Part model, mm, in its own coordinate system. A direction names the side the tool comes from. Round coordinates to 2 decimals unless told otherwise and drop trailing zeros. Write each loop counter-clockwise with the first axis right and the second up, starting at its lowest first coordinate (ties: lowest second). Pieces come first, ordered by that corner, then holes. Notation, with made-up numbers: M -19.75,10 L 17.25,10 A12 cw 17.25,15 Z; hole C -32.5,35.25 d8. An arc over 180 degrees is marked long. One line per question, with ' | ' between items. Start each with the question number.
1) Saw through at C-C (z = -25). List the corners of the cut face in (x, y).
2) Saw through at A-A (z = 26). List the corners of the cut face in (x, y).
3) Wall check: probe 1 along Z at (x, y) = (2.2, 122); probe 2 along Z at (x, y) = (3.35, -122); probe 3 along Y at (x, z) = (4.1, 38.71). Give the ranges that are in metal, low to high. Write a range as [from, to].
4) Drop flat-ended pins along their axis: pin 1 Ø3 at (x, z) = (3, 23.5) entering from +Y; pin 2 Ø1.5 at (x, y) = (0.5, -40) entering from -Z; pin 3 Ø1.8 at (x, z) = (2, -54.5) entering from -Y. Give the stop position or say it passes through.
5) Tool access for faces 4 (the face through (3, 13, -29.205)), 5 (the face through (3, 119, 47)), 6 (the face through (3, 89, -53)): list every direction of +Z, -Z, +X, -X, +Y, -Y with a clear straight run to the whole face (end or side of a thin tool).
6) Saw through at B-B (x = 3.35). Give the number of separate pieces and of enclosed holes in the cut face, plus the area to 3 significant figures.
7) Mould opens along Z. For faces 1 (the face through (3, -69, -53)), 2 (the face through (3, -49, -50.29)), 3 (the face through (3, -122, -6)) say: pulls with the +Z half, pulls with the -Z half, needs draft (parallel to the pull), parting line crosses it, or undercut.
8) Saw through at D-D (y = 98). List the corners of the cut face in (x, z).
```python
from build123d import *

# Parameters (mm, degrees)
ESQUISSE1_W             = 100.58
ESQUISSE1_H             = 238
ESQUISSE1_W_2           = 10
ESQUISSE1_H_2           = 6
ESQUISSE1_W_3           = 15
BOSS_EXTRU_1_DEPTH      = 6
ESQUISSE3_W             = 20
ESQUISSE3_H             = 6
ESQUISSE3_W_2           = 6
ESQUISSE3_H_2           = 20
ESQUISSE3_W_3           = 10
BOSS_EXTRU_5_DEPTH      = 6
ESQUISSE7_W             = 6.88
ESQUISSE7_H             = 7
ENL_V_MAT_EXTRU_3_DEPTH = 6
ESQUISSE8_R             = 1.5
ENL_V_MAT_EXTRU_4_DEPTH = 6


with BuildPart() as part:
    # Esquisse1 → Boss.-Extru.1 (new body)
    with BuildSketch(Plane(origin=(0, 0, 0), x_dir=(0, 0, -1), z_dir=(1, 0, 0))):
        Rectangle(ESQUISSE1_W, ESQUISSE1_H)
        with Locations((-36.29, -51)):
            Rectangle(ESQUISSE1_W_2, ESQUISSE1_H_2, mode=Mode.SUBTRACT)
        with Locations((-23.295, 13)):
            Rectangle(ESQUISSE1_W_3, ESQUISSE1_H_2, mode=Mode.SUBTRACT)
        with Locations((21.705, 13)):
            Rectangle(ESQUISSE1_W_3, ESQUISSE1_H_2, mode=Mode.SUBTRACT)
    extrude(amount=BOSS_EXTRU_1_DEPTH)

    # Esquisse3 → Boss.-Extru.5 (add)
    with BuildSketch(Plane(origin=(6, 0, 0), x_dir=(0, 0, -1), z_dir=(1, 0, 0))):
        with Locations((-40.29, -122)):
            Rectangle(ESQUISSE3_W, ESQUISSE3_H)
        with Locations((32.29, -122)):
            Rectangle(ESQUISSE3_W, ESQUISSE3_H)
        with Locations((53.29, 19)):
            Rectangle(ESQUISSE3_W_2, ESQUISSE3_H_2)
        with Locations((53.29, 79)):
            Rectangle(ESQUISSE3_W_2, ESQUISSE3_H_2)
        with Locations((53.29, -79)):
            Rectangle(ESQUISSE3_W_2, ESQUISSE3_H_2)
        with Locations((53.29, -19)):
            Rectangle(ESQUISSE3_W_2, ESQUISSE3_H_2)
        with Locations((-4, -122)):
            Rectangle(ESQUISSE3_W, ESQUISSE3_H)
        with Locations((33.41, 122)):
            Rectangle(ESQUISSE3_W_3, ESQUISSE3_H)
        with Locations((-38.71, 122)):
            Rectangle(ESQUISSE3_W_3, ESQUISSE3_H)
    extrude(amount=-BOSS_EXTRU_5_DEPTH)

    # Esquisse7 → Enlèv. mat.-Extru.3 (cut)
    with BuildSketch(Plane.ZY):
        with Locations((-46.85, 115.5)):
            Rectangle(ESQUISSE7_W, ESQUISSE7_H)
    extrude(amount=-ENL_V_MAT_EXTRU_3_DEPTH, mode=Mode.SUBTRACT)

    # Esquisse8 → Enlèv. mat.-Extru.4 (cut)
    with BuildSketch(Plane.ZY):
        with Locations((4, -122)):
            Circle(ESQUISSE8_R)
        with Locations((-9.205, 13)):
            Circle(ESQUISSE8_R)
        with Locations((10.795, 13)):
            Circle(ESQUISSE8_R)
        with Locations((45.08, -51)):
            Circle(ESQUISSE8_R)
        with Locations((38.71, 122)):
            Circle(ESQUISSE8_R)
        with Locations((-33.41, 122)):
            Circle(ESQUISSE8_R)
        with Locations((40.29, -122)):
            Circle(ESQUISSE8_R)
        with Locations((-53.29, 79)):
            Circle(ESQUISSE8_R)
        with Locations((-32.29, -122)):
            Circle(ESQUISSE8_R)
        with Locations((-53.29, 19)):
            Circle(ESQUISSE8_R)
        with Locations((-53.29, -79)):
            Circle(ESQUISSE8_R)
        with Locations((-53.29, -19)):
            Circle(ESQUISSE8_R)
    extrude(amount=-ENL_V_MAT_EXTRU_4_DEPTH, mode=Mode.SUBTRACT)


solid = part.part
```
Answer key:
1) outline: M 0,-125 L 6,-125 L 6,10 L 0,10 Z; M 0,16 L 6,16 L 6,119 L 0,119 Z
2) outline: M 0,-119 L 6,-119 L 6,10 L 0,10 Z; M 0,16 L 6,16 L 6,119 L 0,119 Z
3) probe 1: z = [-38.41, -34.91], [-31.91, -28.41], [33.71, 37.21], [40.21, 43.71] | probe 2: z = [-42.29, -33.79], [-30.79, -22.29], [-6, 2.5], [5.5, 14], [30.29, 38.79], [41.79, 50.29] | probe 3: y = [-125, -54], [-48, 120.5], [123.5, 125]
4) pin 1: stops at y = 119 | pin 2: stops at z = -50.29 | pin 3: stops at y = -89
5) face 4: +X, -X | face 5: +Z, +X, -X, +Y | face 6: -Z, +X, -X, +Y
6) separate pieces: 1 | enclosed holes: 15 | area: 24,500 mm2
7) face 1: needs draft | face 2: pulls with the -Z half | face 3: undercut
8) outline: M 0,-50.29 L 6,-50.29 L 6,50.29 L 0,50.29 Z
